Geometry check sheet. Reference: the model listing, model coordinates, mm. A direction names the side the tool comes from. Coordinates: 2 decimals unless noted, no trailing zeros. Write each loop counter-clockwise with the first axis right and the second up, starting at its lowest first coordinate (ties: lowest second). Pieces come first, ordered by that corner, then holes. Notation, with made-up numbers: M 34,7.25 L 60,7.25 A6 ccw 60,12.25 Z; hole C -18.75,-12.75 d10. An arc over 180 degrees is marked long. Put each result on its own line as item: value. Start each with the question number.
1) Scan lines: line 1 along Z through (x, y) = (-4, 76); line 2 along Y through (x, z) = (12, 45) (3 decimals); line 3 along X through (y, z) = (73.5, 69). Record each from-to range of solid material in increasing order.
2) Mould release check, pull along Y, two halves, no side actions. Record for faces 1 (the cylindrical face through (-9.984, -95.561, 38.633)), 2 (the flat face through (-36, 8, 0)), 3 (the cylindrical face through (-6.439, -85.285, 40.961)): released by +Y, released by -Y, zero draft, split by the parting line, or undercut.
3) Cross-section at D-D on z = 56.5. Record the cut outline in (x, y) (3 decimals), plus the area to 3 significant figures.
4) Set-up check for faces 4 (the cylindrical face through (16.19, -91.99, 2.72)), 5 (the flat face through (9, 85.725, 38)), 6 (the flat face through (-12.7, -66, 38)): record each of +Z, -Z, +X, -X, +Y, -Y from which the full face is reachable in a straight line by a thin tool's end or side.
5) Cross-section at C-C on z = 30.5. Record the cut outline in (x, y) (3 decimals).
6) Cross-section at B-B on y = -76.2. Record the cut outline in (x, z) (3 decimals), plus the area to 3 significant figures.
7) Gauge pin test, flat ends, axial feed: pin 1 (2 mm diameter, centred on y = 38.5, z = 61, fed in from +X); pin 2 (8 mm diameter, centred on y = 47, z = 67.5, fed in from -X); pin 3 (18 mm diameter, centred on y = 70, z = 33, fed in from -X); pin 4 (15 mm diameter, centred on y = -76.2, z = 38.1, fed in from -X). Record the tip position at first contact, or that the pin passes through.
8) Cross-section at A-A on x = 5. Record the cut outline in (y, z) (3 decimals), plus the area to 3 significant figures.
from build123d import *

# Parameters (mm, degrees)
F1_DEPTH = 76.2
F2_R     = 9.525
F3_DEPTH = 25.4
F4_R     = 9.525


with BuildPart() as f1:
    # F0 (on Top) → F1 (new body)
    with BuildSketch(Plane.XY):
        with BuildLine():
            ThreePointArc((0, -34.925), (-34.925, 0), (0, 34.925))
            Line((0, 34.925), (0, 47.625))
            Line((0, 47.625), (0, 56.876238))
            Line((0, 56.876238), (0, 85.725))
            Line((0, 85.725), (19.05, 85.725))
            Line((19.05, 85.725), (19.05, 98.425))
            Line((19.05, 98.425), (-12.7, 98.425))
            Line((-12.7, 98.425), (-12.7, 45.900443))
            ThreePointArc((-12.7, 45.900443), (-47.625, 0), (-12.7, -45.900443))
            Line((-12.7, -45.900443), (-12.7, -98.425))
            Line((-12.7, -98.425), (19.05, -98.425))
            Line((19.05, -98.425), (19.05, -85.725))
            Line((19.05, -85.725), (0, -85.725))
            Line((0, -85.725), (0, -47.625))
            Line((0, -47.625), (0, -34.925))
        make_face()
    extrude(amount=F1_DEPTH)

    # F2 (on face) → F3 (cut)
    with BuildSketch(Plane(origin=(-12.7, 0, 0), x_dir=(0, -1, 0), z_dir=(-1, 0, 0))):
        with Locations((-76.2, 38.1)):
            Circle(F2_R)
        with Locations((76.2, 38.1)):
            Circle(F2_R)
    extrude(amount=-F3_DEPTH, mode=Mode.SUBTRACT)

    # F4
    f4_edges = [f1.edges().sort_by_distance(p)[0] for p in [
        (-12.7, -45.900443, 38.1),
        (-12.7, 45.900443, 38.1),
        (-12.7, 98.425, 38.1),
        (-12.7, -98.425, 38.1),
        (19.05, -92.075, 0),
        (19.05, 92.075, 0),
        (19.05, 92.075, 76.2),
        (19.05, -92.075, 76.2),
    ]]
    fillet(f4_edges, radius=F4_R)


solid = f1.part
Answer key:
1. line 1: z = 0 to 28.58, 47.62 to 76.2
1. line 2: y = -98.425 to -85.725, 85.725 to 98.425
1. line 3: x = -12.7 to 0
2. face 1: released by -Y
2. face 2: zero draft
2. face 3: undercut
3. outline: M -18.521,-43.876 A9.525 cw -12.7,-52.651 L -12.7,-88.9 A9.525 ccw -3.175,-98.425 L 19.05,-98.425 L 19.05,-85.725 L 0,-85.725 L 0,-34.925 A34.925 cw 0,34.925 L 0,85.725 L 19.05,85.725 L 19.05,98.425 L -3.175,98.425 A9.525 ccw -12.7,88.9 L -12.7,52.651 A9.525 cw -18.521,43.876 A47.625 ccw Z
3. area: 3,410 mm²
4. face 4: -Z, +X, +Y, -Y
4. face 5: +Z, -Z, +X
4. face 6: +Z, -Z, -X, -Y
5. outline: M -18.521,-43.876 A9.525 cw -12.7,-52.651 L -12.7,-70.458 L 0,-70.458 L 0,-34.925 A34.925 cw 0,34.925 L 0,70.458 L -12.7,70.458 L -12.7,52.651 A9.525 cw -18.521,43.876 A47.625 ccw Z; M -12.7,-88.9 A9.525 ccw -3.175,-98.425 L 19.05,-98.425 L 19.05,-85.725 L 0,-85.725 L 0,-81.942 L -12.7,-81.942 Z; M -12.7,81.942 L 0,81.942 L 0,85.725 L 19.05,85.725 L 19.05,98.425 L -3.175,98.425 A9.525 ccw -12.7,88.9 Z
6. outline: M -12.7,0 L 0,0 L 0,28.575 L -12.7,28.575 Z; M -12.7,47.625 L 0,47.625 L 0,76.2 L -12.7,76.2 Z
6. area: 726 mm²
7. pin 1: stops at x = 0
7. pin 2: stops at x = -20.47
7. pin 3: stops at x = -12.7
7. pin 4: passes through
8. outline: M -98.425,0 L -85.725,0 L -85.725,76.2 L -98.425,76.2 Z; M 85.725,0 L 98.425,0 L 98.425,76.2 L 85.725,76.2 Z
8. area: 1,940 mm²
